from build123d import *

# Parameters (mm, degrees)
BOSS_EXTRUDE1_DEPTH = 15
FILLET1_R           = 20
FILLET2_R           = 5
FILLET3_R           = 50


with BuildPart() as part:
    # Sketch1 → Boss-Extrude1 (new body)
    # profile 1 of 2: a face of its own
    with BuildSketch(Plane.XY):
        with BuildLine():
            Line((0, 0), (5, 0))
            Line((5, 0), (10, 0))
            Line((10, 0), (10, 40))
            ThreePointArc((10, 40), (-6.618184888, 66.911601725), (-4.062833515, 98.437282617))
            Line((-4.062833515, 98.437282617), (-12.996544728, 129.388331338))
            Line((-12.996544728, 129.388331338), (-15.666737168, 138.639274683))
            ThreePointArc((-15.666737168, 138.639274683), (-23.995534595, 84.376466953), (0, 35))
            Line((0, 35), (0, 25))
            Line((0, 25), (0, 0))
        make_face()
        with BuildLine():
            ThreePointArc((7, 5), (6.414213562, 3.585786438), (5, 3))
            ThreePointArc((5, 3), (3, 5), (5, 7))
            ThreePointArc((5, 7), (6.414213562, 6.414213562), (7, 5))
        make_face(mode=Mode.SUBTRACT)
        with BuildLine():
            ThreePointArc((7, 35), (6.414213562, 33.585786438), (5, 33))
            ThreePointArc((5, 33), (3, 35), (5, 37))
            ThreePointArc((5, 37), (6.414213562, 36.414213562), (7, 35))
        make_face(mode=Mode.SUBTRACT)
    # profile 2 of 2: a face of its own
    with BuildSketch(Plane.XY):
        with BuildLine():
            Line((0, 0), (5, 0))
            Line((5, 0), (10, 0))
            Line((10, 0), (10, 40))
            ThreePointArc((10, 40), (-6.618184888, 66.911601725), (-4.062833515, 98.437282617))
            Line((-4.062833515, 98.437282617), (-12.996544728, 129.388331338))
            Line((-12.996544728, 129.388331338), (-15.666737168, 138.639274683))
            ThreePointArc((-15.666737168, 138.639274683), (-23.995534595, 84.376466953), (0, 35))
            Line((0, 35), (0, 25))
            Line((0, 25), (0, 0))
        make_face()
        with BuildLine():
            ThreePointArc((7, 5), (6.414213562, 3.585786438), (5, 3))
            ThreePointArc((5, 3), (3, 5), (5, 7))
            ThreePointArc((5, 7), (6.414213562, 6.414213562), (7, 5))
        make_face(mode=Mode.SUBTRACT)
        with BuildLine():
            ThreePointArc((7, 35), (6.414213562, 33.585786438), (5, 33))
            ThreePointArc((5, 33), (3, 35), (5, 37))
            ThreePointArc((5, 37), (6.414213562, 36.414213562), (7, 35))
        make_face(mode=Mode.SUBTRACT)
    extrude(amount=BOSS_EXTRUDE1_DEPTH)

    # Fillet1
    fillet1_edges = [part.edges().sort_by_distance(p)[0] for p in [
        (10, 40, 7.5),
    ]]
    fillet(fillet1_edges, radius=FILLET1_R)

    # Fillet2
    fillet2_edges = [part.edges().sort_by_distance(p)[0] for p in [
        (0, 0, 7.5),
        (10, 0, 7.5),
    ]]
    fillet(fillet2_edges, radius=FILLET2_R - 0.0001)  # a hair under: the kernel refuses the full size

    # Fillet3
    fillet3_edges = [part.edges().sort_by_distance(p)[0] for p in [
        (0, 35, 7.5),
    ]]
    fillet(fillet3_edges, radius=FILLET3_R)


solid = part.part
The listing builds one solid part. Answer for the finished solid, in the listing's coordinates (mm). A direction names the side the tool comes from. Round coordinates to 2 decimals unless told otherwise and drop trailing zeros. Loops run counter-clockwise (first coordinate to the right, second up) from the corner with the lowest first, then second, coordinate; pieces in that order, holes last. Notation, with made-up numbers: M 49.5,85.25 L 108.5,85.25 A25 ccw 108.5,104.25 Z; hole C -24.75,41.5 d2. An arc over 180 degrees is marked long. Write each question's results on one line, items separated by ' | '. Start each with the question number.
1) Find section A-A on z = 13.5. Count the separate pieces of the cut face and the enclosed holes in it, plus the area to 3 significant figures.
2) Find section C-C on x = -19.5. Write down the section's boundary in (y, z).
3) Straight lines are drawn through the part: probe 1 along X at (y, z) = (34, 2.5); probe 2 along Y at (x, z) = (3.5, 14); probe 3 along X at (y, z) = (36, 9.5). For each, find the intervals that lie inside material, in ascending order.
4) Which of the six approach directions +Z, -Z, +X, -X, +Y, -Y give full straight-line access (tool end or side, diameter ignored) to faces 5 (the flat face through (-8, 70, 15)), 6 (the flat face through (0, 11, 7))?
5) Each of these flat-tipped pins is pushed along its axis until it touches: pin 1 (4 mm diameter, centred on y = 60, z = 5, fed in from +X); pin 2 (4 mm diameter, centred on x = 1, z = 12.5, fed in from -Y); pin 3 (6 mm diameter, centred on y = 35, z = 6.5, fed in from -X). Where does it stop, or does it pass through?
6) Find section B-B on y = 108.5. Write down the section's boundary in (x, z).
7) Determine the mould class of faces 1 (the cylindrical face through (-24.827, 92.03, 7.395)), 2 (the cylindrical face through (-7.26, 70, 7.4)), 3 (the flat face through (-8, 70, 0)), 4 (the cylindrical face through (9, 2, 8)) for opening direction Y: pulls with the +Y half, pulls with the -Y half, needs draft (parallel to the pull), parting line crosses it, or undercut.
Final values:
1) separate pieces: 1 | enclosed holes: 2 | area: 1,730 mm²
2) outline: M 66.7,0 L 129.61,0 L 129.61,15 L 66.7,15 Z
3) probe 1: -2.77 to 3.27, 6.73 to 9.86 | probe 2: 0.23 to 3.68, 6.32 to 33.68, 36.32 to 46.58 | probe 3: -3.51 to 3.27, 6.73 to 9.51
4) face 5: +Z, +X, -X, +Y, -Y | face 6: +Z, -Z, -X, -Y
5) pin 1: x = -3.57 | pin 2: y = 0.42 | pin 3: x = -4.36
6) outline: M -24.45,0 L -6.97,0 L -6.97,15 L -24.45,15 Z
7) face 1: parting line crosses it | face 2: undercut | face 3: needs draft | face 4: pulls with the -Y half
